Drawing for the job (mm, zero at the part's lowest x, y, z). A direction names the side the tool comes from. Round coordinates to 2 decimals unless told otherwise and drop trailing zeros. Write each loop counter-clockwise with the first axis right and the second up, starting at its lowest first coordinate (ties: lowest second). Pieces come first, ordered by that corner, then holes. Notation, with made-up numbers: M 1.25,-21 L 39.25,-21 A10 cw 39.25,-5 Z; hole C 14,86 d1. An arc over 180 degrees is marked long. Use a Markdown table: item, result. Add a question column.
1) Which spindle directions (+Z, -Z, +X, -X, +Y, -Y) get a long thin tool onto all of the face, cutting with end or side? Do the marked faces 4 and 5. Say none if no direction does.
2) Slice it at B-B on x = 82.4. Write the cut outline in (y, z).
3) Two-plate mould, pull along Y, no slides. Class the marked faces 1, 2 and 3: released by +Y, released by -Y, zero draft, split by the parting line, or undercut.
4) Wall check: probe 1 along Y at (x, z) = (82.4, 7.75); probe 2 along X at (y, z) = (25.5, 4.75); probe 3 along X at (y, z) = (27, 7). Give the ranges that are in metal, low to high.
5) Slice it at A-A on y = 28. Write the cut outline in (x, z).
6) Slice it at C-C on z = 2.75. Give the number of separate pieces and of enclosed holes in the cut face, plus the area to 3 significant figures.
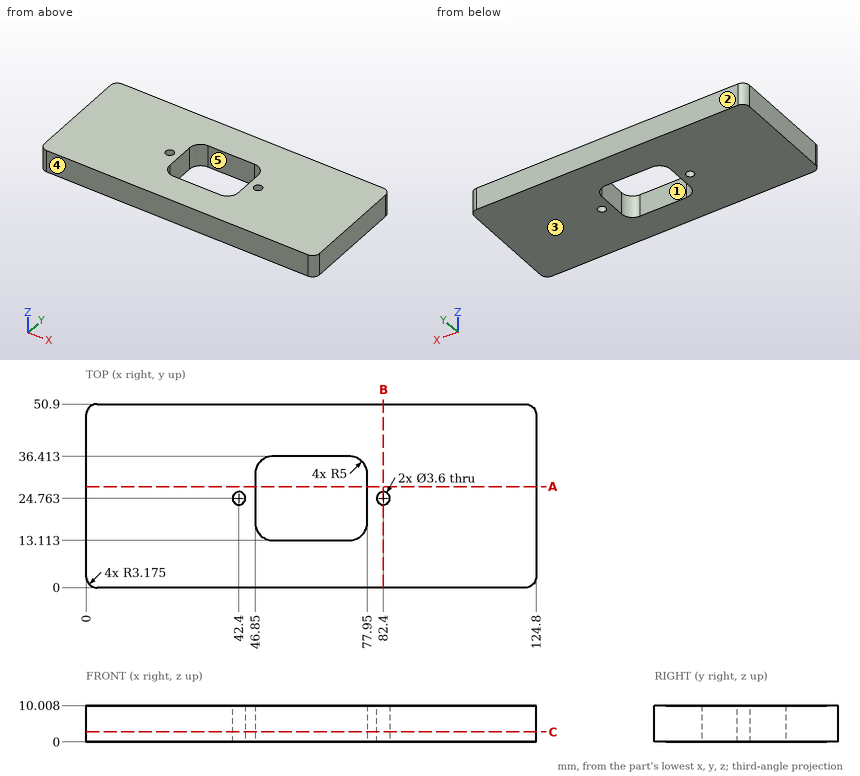
Entries:
| question | item | result |
|---|---|---|
| 1 | face 4 | +Z, -Z, +X, -X, -Y |
| 1 | face 5 | +Z, -Z |
| 2 | outline | M 0,0 L 22.96,0 L 22.96,10.01 L 0,10.01 Z; M 26.56,0 L 50.9,0 L 50.9,10.01 L 26.56,10.01 Z |
| 3 | face 1 | undercut |
| 3 | face 2 | released by +Y |
| 3 | face 3 | zero draft |
| 4 | probe 1 | y = 0 to 22.96, 26.56 to 50.9 |
| 4 | probe 2 | x = 0 to 40.76, 44.04 to 46.85, 77.95 to 80.76, 84.04 to 124.8 |
| 4 | probe 3 | x = 0 to 46.85, 77.95 to 124.8 |
| 5 | outline | M 0,0 L 46.85,0 L 46.85,10.01 L 0,10.01 Z; M 77.95,0 L 124.8,0 L 124.8,10.01 L 77.95,10.01 Z |
| 6 | separate pieces | 1 |
| 6 | enclosed holes | 3 |
| 6 | area | 5,620 mm^2 |
